The figure shows three views and two pictorial views of one solid part (mm, origin at its lowest corner). Answer the questions. A direction names the side the tool comes from. Round coordinates to 2 decimals unless told otherwise and drop trailing zeros. Write each loop counter-clockwise with the first axis right and the second up, starting at its lowest first coordinate (ties: lowest second). Pieces come first, ordered by that corner, then holes. Notation, with made-up numbers: M 63,64.25 L 118,64.25 A21 ccw 118,89.25 Z; hole C 3,62.5 d10. An arc over 180 degrees is marked long. One line per item, written item: value. Start each with the question number.
Q1. A tool of negligible diameter and unlimited length cuts with its end or side. For the marked faces 4, 5 and 6, from which of +Z, -Z, +X, -X, +Y, -Y can it reach the whole face along a straight path? Write none if from no direction.
Q2. The mould has two halves that part along X. Classify the marked faces 1, 2 and 3: released by +X, released by -X, zero draft, split by the parting line, or undercut.
Q3. Consider probe 1 along X at (y, z) = (0.9, 10); probe 2 along Y at (x, z) = (13, 11.5); probe 3 along X at (y, z) = (4.6, 4). Determine where each line is inside the solid, lowest interval first.
Q4. Find section A-A (x = 10). Count the separate pieces of the cut face and the enclosed holes in it, and give its area (3 significant figures).
Q5. Find section C-C (y = 6.5). Write down the section's boundary in (x, z).
Q6. Given pin 1 Ø2.5 at (x, z) = (10, 3) entering from +Y; pin 2 Ø6 at (x, z) = (3, 14) entering from +Y; pin 3 Ø3 at (x, z) = (11, 11) entering from -Y, each flat-ended and moving along its own axis, determine where each tip first touches the part or whether it passes through.
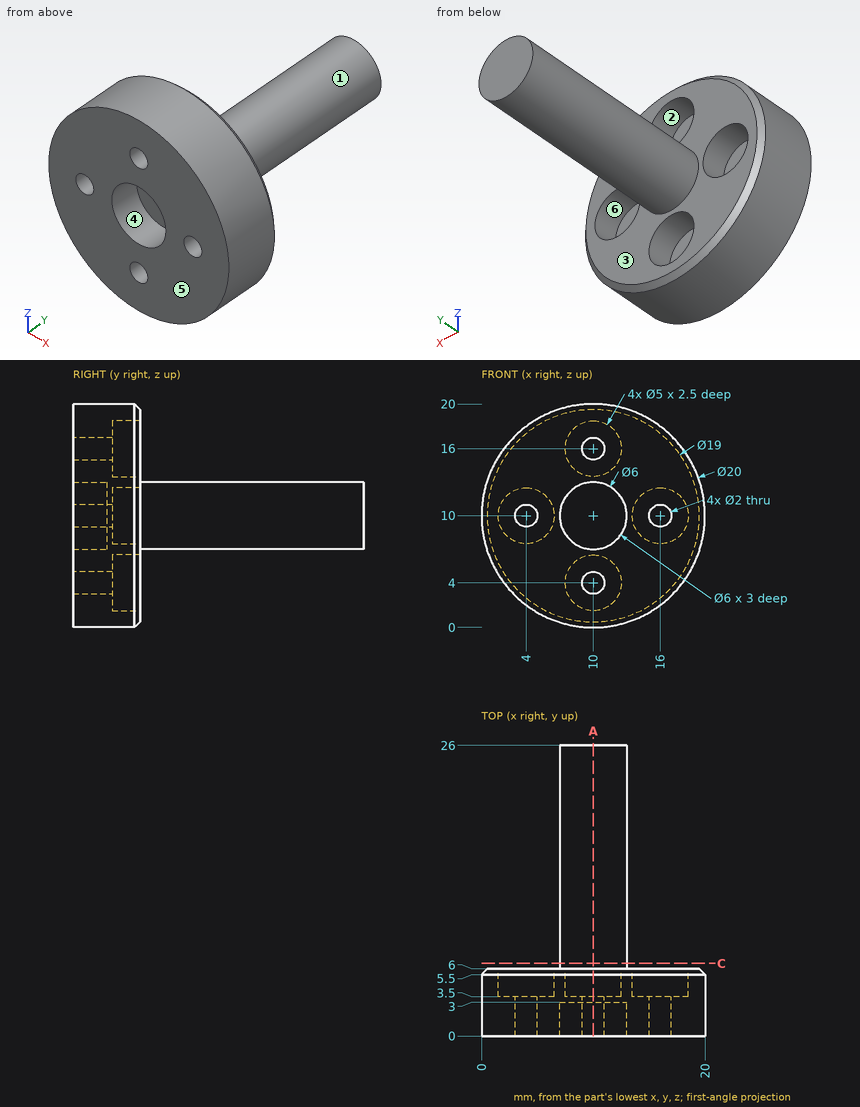
The answers:
1. face 4: -Y
1. face 5: +Z, -Z, +X, -X, -Y
1. face 6: +Y
2. face 1: split by the parting line
2. face 2: undercut
2. face 3: zero draft
3. probe 1: 0 to 3, 5 to 7, 13 to 15, 17 to 20
3. probe 2: 0 to 6
3. probe 3: 2 to 7.5, 12.5 to 18
4. separate pieces: 3
4. enclosed holes: 0
4. area: 183 mm2
5. outline: C 10,10 d6
6. pin 1: y = 3.5
6. pin 2: y = 6
6. pin 3: y = 3
